```python
from build123d import *

# Parameters (mm, degrees)
SKIZZE1_R                       = 50
AUFSATZ_LINEAR_AUSTRAGEN1_DEPTH = 10
SKIZZE2_R                       = 3
SCHNITT_LINEAR_AUSTRAGEN2_DEPTH = 10
SKIZZE3_R                       = 30
AUFSATZ_LINEAR_AUSTRAGEN2_DEPTH = 78.6
VERRUNDUNG1_R                   = 2
FASE1_SIZE                      = 1
SKIZZE4_R                       = 22.5
AUFSATZ_LINEAR_AUSTRAGEN3_DEPTH = 24.9
SKIZZE5_R                       = 21.25
AUFSATZ_LINEAR_AUSTRAGEN4_DEPTH = 1.85
SKIZZE6_R                       = 22.5
AUFSATZ_LINEAR_AUSTRAGEN5_DEPTH = 13.25
FASE2_SIZE                      = 1.5
SKIZZE7_R                       = 20
AUFSATZ_LINEAR_AUSTRAGEN6_DEPTH = 45
FASE3_SIZE                      = 1.5
SKIZZE8_R                       = 30
AUFSATZ_LINEAR_AUSTRAGEN7_DEPTH = 20
FASE4_SIZE                      = 1
VERRUNDUNG2_R                   = 2
FASE5_SIZE                      = 0.5
FASE6_SIZE                      = 0.5
SKIZZE9_R                       = 27.5
AUFSATZ_LINEAR_AUSTRAGEN8_DEPTH = 138
SKIZZE10_R                      = 22.5
AUFSATZ_LINEAR_AUSTRAGEN9_DEPTH = 45
VERRUNDUNG3_R                   = 1
FASE7_SIZE                      = 1
VERRUNDUNG4_R                   = 1
FASE8_SIZE                      = 1.5


with BuildPart() as part:
    # Skizze1 → Aufsatz-Linear austragen1 (new body)
    with BuildSketch(Plane(origin=(0, 0, 0), x_dir=(1, 0, 0), z_dir=(0, 1, 0))):
        with Locations(Location((0, 0, 0), (0, 0, 270))):  # turned: the seam where the file's is
            Circle(SKIZZE1_R)
    extrude(amount=AUFSATZ_LINEAR_AUSTRAGEN1_DEPTH)

    # Skizze2 → Schnitt-Linear austragen2 (cut)
    with BuildSketch(Plane(origin=(0, 10, 0), x_dir=(1, 0, 0), z_dir=(0, 1, 0))):
        with Locations(Location((-33.169696769, 24.099195344, 0), (0, 0, 270))):  # turned: the seam where the file's is
            Circle(SKIZZE2_R)
        with Locations(Location((33.169696769, 24.099195344, 0), (0, 0, 270))):  # turned: the seam where the file's is
            Circle(SKIZZE2_R)
        with Locations(Location((12.669696769, 38.993317168, 0), (0, 0, 270))):  # turned: the seam where the file's is
            Circle(SKIZZE2_R)
        with Locations(Location((41, 0, 0), (0, 0, 270))):  # turned: the seam where the file's is
            Circle(SKIZZE2_R)
        with Locations(Location((33.169696769, -24.099195344, 0), (0, 0, 270))):  # turned: the seam where the file's is
            Circle(SKIZZE2_R)
        with Locations(Location((12.669696769, -38.993317168, 0), (0, 0, 270))):  # turned: the seam where the file's is
            Circle(SKIZZE2_R)
        with Locations(Location((-12.669696769, -38.993317168, 0), (0, 0, 270))):  # turned: the seam where the file's is
            Circle(SKIZZE2_R)
        with Locations(Location((-33.169696769, -24.099195344, 0), (0, 0, 270))):  # turned: the seam where the file's is
            Circle(SKIZZE2_R)
        with Locations(Location((-41, 0, 0), (0, 0, 270))):  # turned: the seam where the file's is
            Circle(SKIZZE2_R)
        with Locations(Location((-12.669696769, 38.993317168, 0), (0, 0, 270))):  # turned: the seam where the file's is
            Circle(SKIZZE2_R)
    extrude(amount=-SCHNITT_LINEAR_AUSTRAGEN2_DEPTH, mode=Mode.SUBTRACT)

    # Skizze3 → Aufsatz-Linear austragen2 (add)
    with BuildSketch(Plane(origin=(0, 10, 0), x_dir=(1, 0, 0), z_dir=(0, 1, 0))):
        with Locations(Location((0, 0, 0), (0, 0, 270))):  # turned: the seam where the file's is
            Circle(SKIZZE3_R)
    extrude(amount=AUFSATZ_LINEAR_AUSTRAGEN2_DEPTH)

    # Verrundung1
    verrundung1_edges = [part.edges().sort_by_distance(p)[0] for p in [
        (0, 10, -30),
    ]]
    fillet(verrundung1_edges, radius=VERRUNDUNG1_R)

    # Fase1
    fase1_edges = [part.edges().sort_by_distance(p)[0] for p in [
        (0, 88.6, -30),
    ]]
    chamfer(fase1_edges, length=FASE1_SIZE)

    # Skizze4 → Aufsatz-Linear austragen3 (add)
    with BuildSketch(Plane(origin=(0, 88.6, 0), x_dir=(-1, 0, 0), z_dir=(0, 1, 0))):
        with Locations(Location((0, 0, 0), (0, 0, 90))):  # turned: the seam where the file's is
            Circle(SKIZZE4_R)
    extrude(amount=AUFSATZ_LINEAR_AUSTRAGEN3_DEPTH)

    # Skizze5 → Aufsatz-Linear austragen4 (add)
    with BuildSketch(Plane(origin=(0, 113.5, 0), x_dir=(1, 0, 0), z_dir=(0, 1, 0))):
        with Locations(Location((0, 0, 0), (0, 0, 270))):  # turned: the seam where the file's is
            Circle(SKIZZE5_R)
    extrude(amount=AUFSATZ_LINEAR_AUSTRAGEN4_DEPTH)

    # Skizze6 → Aufsatz-Linear austragen5 (add)
    with BuildSketch(Plane(origin=(0, 115.35, 0), x_dir=(1, 0, 0), z_dir=(0, 1, 0))):
        with Locations(Location((0, 0, 0), (0, 0, 270))):  # turned: the seam where the file's is
            Circle(SKIZZE6_R)
    extrude(amount=AUFSATZ_LINEAR_AUSTRAGEN5_DEPTH)

    # Fase2
    fase2_edges = [part.edges().sort_by_distance(p)[0] for p in [
        (0, 128.6, -22.5),
    ]]
    chamfer(fase2_edges, length=FASE2_SIZE)

    # Skizze7 → Aufsatz-Linear austragen6 (add)
    with BuildSketch(Plane(origin=(0, 128.6, 0), x_dir=(1, 0, 0), z_dir=(0, 1, 0))):
        with Locations(Location((0, 0, 0), (0, 0, 270))):  # turned: the seam where the file's is
            Circle(SKIZZE7_R)
    extrude(amount=AUFSATZ_LINEAR_AUSTRAGEN6_DEPTH)

    # Fase3
    fase3_edges = [part.edges().sort_by_distance(p)[0] for p in [
        (0, 173.6, -20),
    ]]
    chamfer(fase3_edges, length=FASE3_SIZE)

    # Skizze8 → Aufsatz-Linear austragen7 (add)
    with BuildSketch(Plane.XZ):
        with Locations(Location((0, 0, 0), (0, 0, 90))):  # turned: the seam where the file's is
            Circle(SKIZZE8_R)
    extrude(amount=AUFSATZ_LINEAR_AUSTRAGEN7_DEPTH)

    # Fase4
    fase4_edges = [part.edges().sort_by_distance(p)[0] for p in [
        (0, -20, -30),
    ]]
    chamfer(fase4_edges, length=FASE4_SIZE)

    # Verrundung2
    verrundung2_edges = [part.edges().sort_by_distance(p)[0] for p in [
        (0, 0, -30),
    ]]
    fillet(verrundung2_edges, radius=VERRUNDUNG2_R)

    # Fase5
    fase5_edges = [part.edges().sort_by_distance(p)[0] for p in [
        (0, 0, -50),
    ]]
    chamfer(fase5_edges, length=FASE5_SIZE)

    # Fase6
    fase6_edges = [part.edges().sort_by_distance(p)[0] for p in [
        (0, 10, -50),
    ]]
    chamfer(fase6_edges, length=FASE6_SIZE)

    # Skizze9 → Aufsatz-Linear austragen8 (add)
    with BuildSketch(Plane.XZ.offset(20)):
        with Locations(Location((0, 0, 0), (0, 0, 270))):  # turned: the seam where the file's is
            Circle(SKIZZE9_R)
    extrude(amount=AUFSATZ_LINEAR_AUSTRAGEN8_DEPTH)

    # Skizze10 → Aufsatz-Linear austragen9 (add)
    with BuildSketch(Plane.XZ.offset(158)):
        with Locations(Location((0, 0, 0), (0, 0, 90))):  # turned: the seam where the file's is
            Circle(SKIZZE10_R)
    extrude(amount=AUFSATZ_LINEAR_AUSTRAGEN9_DEPTH)

    # Verrundung3
    verrundung3_edges = [part.edges().sort_by_distance(p)[0] for p in [
        (0, -20, 27.5),
    ]]
    fillet(verrundung3_edges, radius=VERRUNDUNG3_R)

    # Fase7
    fase7_edges = [part.edges().sort_by_distance(p)[0] for p in [
        (0, -158, 27.5),
    ]]
    chamfer(fase7_edges, length=FASE7_SIZE)

    # Verrundung4
    verrundung4_edges = [part.edges().sort_by_distance(p)[0] for p in [
        (0, -158, -22.5),
    ]]
    fillet(verrundung4_edges, radius=VERRUNDUNG4_R)

    # Fase8
    fase8_edges = [part.edges().sort_by_distance(p)[0] for p in [
        (0, -203, -22.5),
    ]]
    chamfer(fase8_edges, length=FASE8_SIZE)


solid = part.part
```
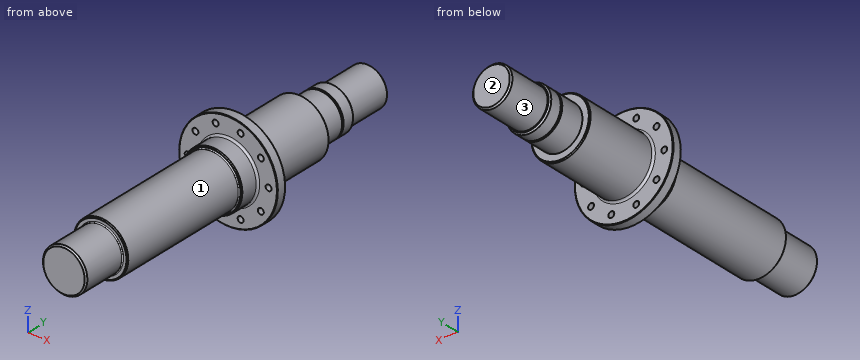
The model under review builds one solid part; all positions refer to its coordinate system, in mm. Face numbers are marked on the shaded views. A direction names the side the tool comes from. Coordinates: 2 decimals unless noted, no trailing zeros. Order: outer loops, then holes, each group sorted by start corner. A loop starts at its lowest first (then second) coordinate and runs counter-clockwise, first axis right, second up. Notation, with made-up numbers: (9.5, 87.5) -> (61.5, 87.5) arc R7 cw to (61.5, 95.5) -> close; hole circle Ø8 at (11.25, 23.5). An arc over 180 degrees is marked (long way). Answer in a Markdown table with one row per item. Add a question column.
Item 1: We need section A-A on y = 51. Write out the cut boundary in (x, z).
Item 2: Clearance check with flat-ended pins moving along their axes: pin 1 (5 mm diameter, centred on x = 26.5, z = -8, fed in from +Y); pin 2 (9.5 mm diameter, centred on x = 41, z = 0, fed in from -Y); pin 3 (5.5 mm diameter, centred on x = 12.67, z = 38.99, fed in from +Y); pin 4 (1.5 mm diameter, centred on x = -6, y = -80, fed in from -Z). State where each tip first meets the part, or that it passes through.
Item 3: To check wall thickness, follow probe 1 along X at (y, z) = (5, 0); probe 2 along Y at (x, z) = (-45, -14); probe 3 along Y at (x, z) = (-19.5, 13). State the ranges of each line that lie inside material, in increasing order.
Item 4: Machinability: for the marked faces 1, 2 and 3, which of the approach directions +Z, -Z, +X, -X, +Y, -Y give a long, thin tool a straight path to every point of the face, cutting with its end or side? Answer none if there is none.
Final values:
| question | item | result |
|---|---|---|
| 1 | outline | circle Ø60 at (0, 0) |
| 2 | pin 1 | stops at y = 88.6 |
| 2 | pin 2 | stops at y = 0 |
| 2 | pin 3 | passes through |
| 2 | pin 4 | stops at z = -26.99 |
| 3 | probe 1 | x = -50 to -44, -38 to 38, 44 to 50 |
| 3 | probe 2 | y = 0 to 10 |
| 3 | probe 3 | y = -158 to 88.6 |
| 4 | face 1 | -Y |
| 4 | face 2 | +Z, -Z, +X, -X, +Y |
| 4 | face 3 | +Y |
